Read the model definition and answer for the solid it produces. Units are mm, in the model's axes. Round coordinates to 2 decimals unless told otherwise and drop trailing zeros. Order: outer loops, then holes, each group sorted by start corner. A loop starts at its lowest first (then second) coordinate and runs counter-clockwise, first axis right, second up.
from build123d import *

# Parameters (mm, degrees)
BOSS_EXTRUDE1_DEPTH     = 708.025
FILLET1_R               = 2.54
F_1_4_CLEARANCE_HOLE1_D = 6.7564
LPATTERN1_COUNT         = 6
LPATTERN1_PITCH         = 266.7
F_1_4_CLEARANCE_HOLE4_D = 6.7564
LPATTERN4_COUNT         = 6
LPATTERN4_PITCH         = 266.7


with BuildPart() as part:
    # Sketch1 → Boss-Extrude1 (new, symmetric)
    with BuildSketch(Plane.XY):
        Polygon((0, 0), (0, 50.8), (4.7625, 50.8), (4.7625, 4.7625), (50.8, 4.7625), (50.8, 0), align=None)
    extrude(amount=BOSS_EXTRUDE1_DEPTH, both=True)

    # Fillet1
    fillet1_edges = [part.edges().sort_by_distance(p)[0] for p in [
        (4.7625, 50.8, 0),
        (4.7625, 4.7625, 0),
        (50.8, 4.7625, 0),
    ]]
    fillet(fillet1_edges, radius=FILLET1_R)

    # 1/4 Clearance Hole1 (through all)
    with Locations(Plane(origin=(0, 4.7625, 0), x_dir=(1, 0, 0), z_dir=(0, 1, 0))):
        with Locations((14.2875, -679.45), (14.2875, -654.05)):
            f_1_4_clearance_hole1 = Hole(F_1_4_CLEARANCE_HOLE1_D / 2)

    # LPattern1: 1/4 Clearance Hole1 ×6
    with Locations(*[(0, 0, -i * LPATTERN1_PITCH) for i in range(1, LPATTERN1_COUNT)]):
        add(f_1_4_clearance_hole1, mode=Mode.SUBTRACT)

    # 1/4 Clearance Hole4 (through all)
    with Locations(Plane.ZY):
        with Locations((-666.75, 16.66875)):
            f_1_4_clearance_hole4 = Hole(F_1_4_CLEARANCE_HOLE4_D / 2)

    # LPattern4: 1/4 Clearance Hole4 ×6
    with Locations(*[(0, 0, i * LPATTERN4_PITCH) for i in range(1, LPATTERN4_COUNT)]):
        add(f_1_4_clearance_hole4, mode=Mode.SUBTRACT)


solid = part.part
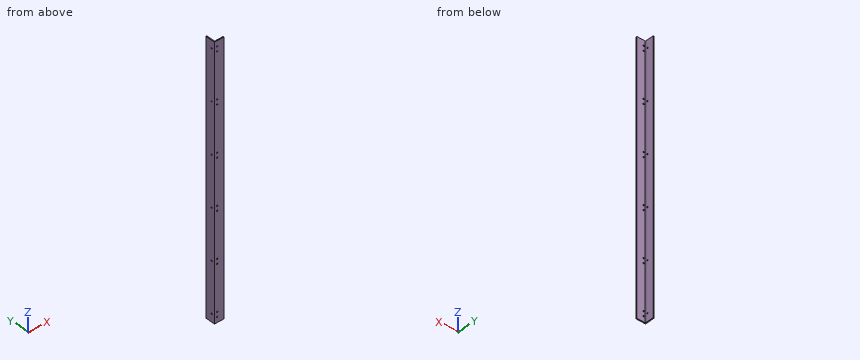
Q1. Straight lines are drawn through the part: probe 1 along Y at (x, z) = (2.7, 666.75); probe 2 along X at (y, z) = (15.5, -645); probe 3 along Y at (x, z) = (3, -133). For each, find the intervals that lie inside material, in ascending order.
Outcome:
probe 1: y = 0 to 13.29, 20.05 to 50.75
probe 2: x = 0 to 4.76
probe 3: y = 0 to 13.31, 20.03 to 50.68
Q2. A cutting plane is placed at A-A, the plane z = 16.5. Give the vertices of the cut face in (x, y).
Outcome:
outline: (0, 0) - (50.8, 0) - (50.8, 2.22) arc R2.54 ccw to (48.26, 4.76) - (7.3, 4.76) arc R2.54 cw to (4.76, 7.3) - (4.76, 48.26) arc R2.54 ccw to (2.22, 50.8) - (0, 50.8) - close
Q3. A cutting plane is placed at B-B, the plane y = 28. Give the vertices of the cut face in (x, z) (1 decimal), plus the area to 3 significant figures.
Outcome:
outline: (0, -708) - (4.8, -708) - (4.8, 708) - (0, 708) - close
area: 6,740 mm2
Q4. Flat-ended cylindrical pins translate along their axes: pin 1 (6 mm diameter, centred on x = 14.29, z = -654.05, fed in from -Y); pin 2 (3 mm diameter, centred on x = 28.5, z = 319.5, fed in from +Y); pin 3 (8 mm diameter, centred on y = 30.5, z = 55.5, fed in from +X); pin 4 (3 mm diameter, centred on y = 6, z = -62.5, fed in from +X). Find the tip coordinate at first contact, or state that the pin passes through.
Outcome:
pin 1: passes through
pin 2: stops at y = 4.76
pin 3: stops at x = 4.76
pin 4: stops at x = 49.38
